Design review of the part built by this model. Coordinates are the model's own, in mm. Face numbers are marked on the shaded views. Coordinates: 2 decimals unless noted, no trailing zeros. Write each loop counter-clockwise with the first axis right and the second up, starting at its lowest first coordinate (ties: lowest second). Pieces come first, ordered by that corner, then holes.
Q1. For L1, parallel to X at y = 3.5, z = -20 (1 decimal); L2, parallel to Z at x = 11, y = 4.5; L3, parallel to X at y = 1.6, z = -3 (1 decimal), list the stretches that pass through material, from the lowest coordinate up.
Q2. Take a section at D-D, the plane y = 2.7. Write out the cut boundary in (x, z) (1 decimal), plus the area to 3 significant figures.
Q3. The part is to be moulded in two halves that separate along X. For the marked faces 1, 2 and 3, say which applies: released by +X, released by -X, zero draft, split by the parting line, or undercut.
Q4. For pin 1 Ø1 at (x, y) = (-1, 0.5) entering from +Z (3 decimals); pin 2 Ø0.6 at (x, y) = (-3, 0.5) entering from -Z; pin 3 Ø2.5 at (x, y) = (-4.5, 3) entering from +Z (3 decimals), all flat-tipped, find the tip position at first contact; note any pin that passes through.
Autodesk Inventor part; units mm, degrees
ref_plane "YZ Plane" through (0, 0, 0) normal (1, 0, 0) x (0, 1, 0)
ref_plane "XZ Plane" through (0, 0, 0) normal (0, 1, 0) x (-1, 0, 0)
ref_plane "XY Plane" through (0, 0, 0) normal (0, 0, 1) x (1, 0, 0)
sketch "Sketch1" plane through (0, 0, 0) normal (0, 1, 0) x (-1, 0, 0)
  line L0 (19.05, 63.5) -> (19.05, -63.5)
  line L1 (19.05, -63.5) -> (-19.05, -63.5)
  line L2 (-19.05, -63.5) -> (-19.05, 63.5)
  line L3 (9.525, 63.5) -> (9.525, -53.975)
  line L4 (9.525, -53.975) -> (-9.525, -53.975)
  line L5 (-9.525, -53.975) -> (-9.525, 63.5)
  line L6 (-19.05, 63.5) -> (-9.525, 63.5)
  line L7 (9.525, 63.5) -> (19.05, 63.5)
  line L8 (-9.525, 41.275) -> (9.525, 41.275)
  line L9 (9.525, 41.275) -> (9.525, 31.75)
  line L10 (9.525, 31.75) -> (-9.525, 31.75)
  line L11 (-9.525, 31.75) -> (-9.525, 41.275)
  point P0 (0, 0)
  dimension "d0" = 38.1
  dimension "d3" = 63.5
  dimension "d4" = 19.05
  dimension "d7" = 9.525
  dimension "d8" = 9.525
  dimension "d10" = 9.525
  dimension "d11" = 127
  dimension "d17" = 9.525
  dimension "d18" = 31.75
extrude "Extrusion2" add sketch "Sketch1" along normal blind 4.7625 contours L0 L1 L2 L6 L5 L4 L3 L7
extrude "Extrusion3" add sketch "Sketch1" along normal blind 1.27 contours L3 L10 L5 L8
chamfer "Chamfer1" distance 4.7625 angle 45 3 edges at (19.05, 4.7625, 0) (-19.05, 4.7625, 0) (0, 4.7625, -63.5)
sketch "Sketch2" plane through (0, 0, 0) normal (1, 0, 0) x (0, 1, 0)
  line L0 (0, -63.5) -> (0, -53.975)
  line L1 (0, -53.975) -> (4.7625, -53.975)
  line L2 (1.27, 31.75) -> (0, 31.75)
  line L3 (0, 31.75) -> (0, 41.275)
  line L4 (0, 41.275) -> (1.27, 41.275)
  line L5 (1.27, 41.275) -> (1.27, 31.75)
  line L6 (1.27, 31.75) -> (0, 31.75)
  line L7 (0, 31.75) -> (0, -53.975)
  line L8 (0, -53.975) -> (4.7625, -53.975)
  line L9 (0, 63.5) -> (4.7625, 63.5)
  line L10 (0, 63.5) -> (0, 41.275)
  line L11 (0, 41.275) -> (1.27, 41.275)
  line L12 (1.27, 41.275) -> (1.27, 31.75)
  circle A0 centre (4.7625, 56.1022) radius 1.27
  circle A1 centre (4.7625, -46.3233) radius 1.27
  line L13 (4.7625, -53.975) -> (4.7625, -58.7375)
  line L14 (4.7625, -58.7375) -> (0, -63.5)
  line L15 (4.7625, 63.5) -> (4.7625, -53.975)
  point P0 (0, 0)
  point P1 (6.35, -57.15)
  point P2 (6.35, -57.15)
  dimension "d24" = 7.3978
  dimension "d25" = 7.6517
  dimension "d26" = 2.54
  dimension "d27" = 4.7625
  dimension "d28" = 4.7625
extrude "Extrusion4" cut sketch "Sketch2" along normal through all both and the other way through all contours L15 A1 | A1 L15 | L15 A0 | A0 L15
equation "\"d8\" = d7"
equation "\"d10\" = d7"
equation "\"d17\" = d7"
equation "\"d12\" = 0.5 * d7"
equation "\"d14\" = 0.5 * d7"
equation "\"d27\" = 0.5 * d7"
equation "\"d28\" = d27"
equation "\"d22\" = 0.75 * d7"
properties part number "LegHolderV4"
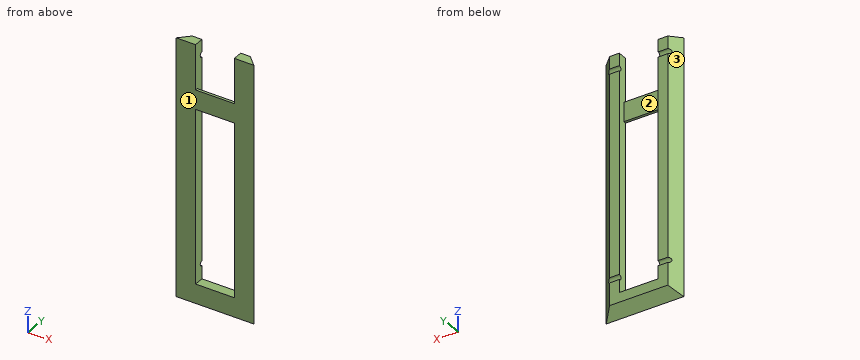
Responses:
1. L1: x = -15.6 to -9.5, 9.5 to 15.6
1. L2: z = -59 to -47.57, -45.08 to 54.86, 57.34 to 63.5
1. L3: x = -17.5 to -9.5, 9.5 to 17.5
2. outline: (-16.4, -60.8) - (16.4, -60.8) - (16.4, 63.5) - (9.5, 63.5) - (9.5, -54) - (-9.5, -54) - (-9.5, 63.5) - (-16.4, 63.5) - close
2. area: 1,830 mm2
3. face 1: zero draft
3. face 2: undercut
3. face 3: released by -X
4. pin 1: stops at z = 41.275
4. pin 2: stops at z = -63.3
4. pin 3: stops at z = -53.975
